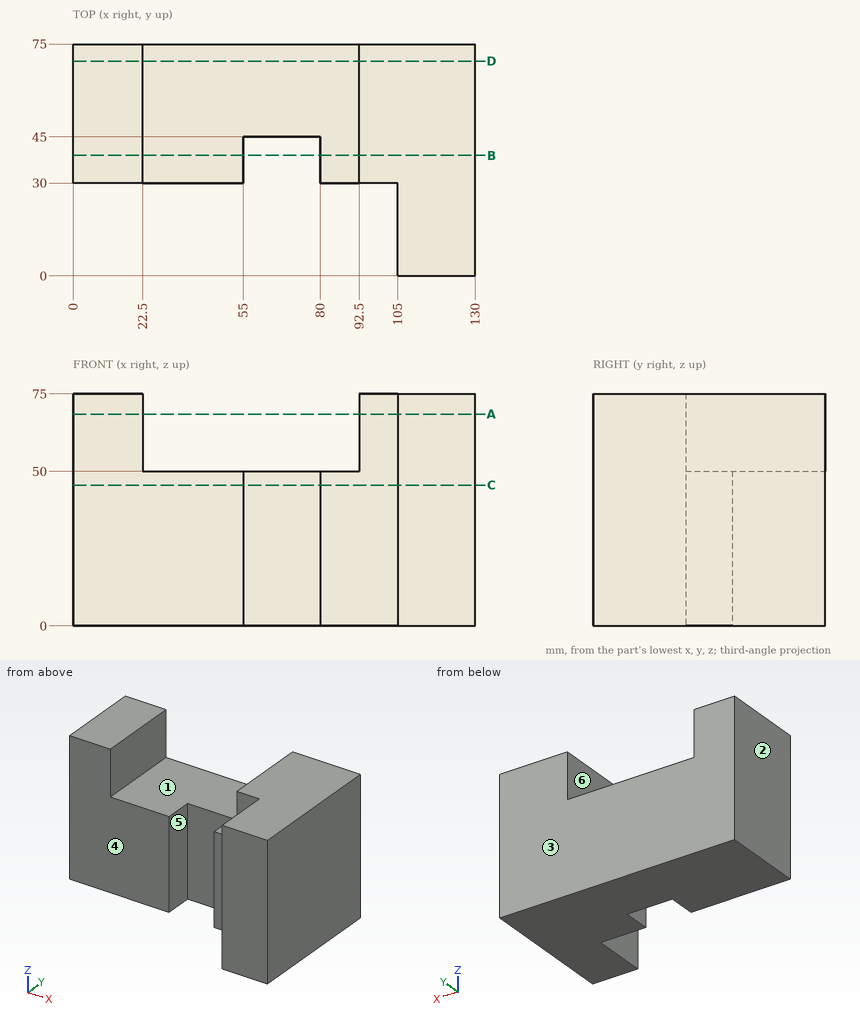
Study the drawing (mm; zero at the part's minimum x, y, z) and answer. A direction names the side the tool comes from. Round coordinates to 2 decimals unless told otherwise and drop trailing zeros. Write each loop counter-clockwise with the first axis right and the second up, starting at its lowest first coordinate (ties: lowest second). Pieces come first, ordered by that corner, then holes. Notation, with made-up numbers: (-29, -9) -> (-5, -9) arc R25 cw to (-5, 16) -> close; hole circle Ø3 at (9.5, -16.5). An arc over 180 degrees is marked (long way). Write each question's results on one line, items separated by ' | '.
Item 1: A cutting plane is placed at C-C, the plane z = 45.5. Determine the outline of the cut face in (x, y), plus the area to 4 significant figures.
Result set:
outline: (0, 30) -> (55, 30) -> (55, 45) -> (80, 45) -> (80, 30) -> (105, 30) -> (105, 0) -> (130, 0) -> (130, 75) -> (0, 75) -> close | area: 6,225 mm^2
Item 2: The mould has two halves that part along X. Classify the marked faces 1, 2 and 3: +X half, -X half, draft (parallel to the pull), parting line (faces both ways), or undercut.
Result set:
face 1: undercut | face 2: -X half | face 3: draft
Item 3: Find the intervals of material crossed by line 1 along X through (y, z) = (47.5, 64.5); line 2 along X through (y, z) = (13.5, 33.5); line 3 along X through (y, z) = (41.5, 34), in increasing order. Write a range as [from, to].
Result set:
line 1: [0, 22.5], [92.5, 130] | line 2: [105, 130] | line 3: [0, 55], [80, 130]
Item 4: A cutting plane is placed at A-A, the plane z = 68.5. Determine the outline of the cut face in (x, y).
Result set:
outline: (0, 30) -> (22.5, 30) -> (22.5, 75) -> (0, 75) -> close; (92.5, 30) -> (105, 30) -> (105, 0) -> (130, 0) -> (130, 75) -> (92.5, 75) -> close
Item 5: Which of the six approach directions +Z, -Z, +X, -X, +Y, -Y give full straight-line access (tool end or side, diameter ignored) to the marked faces 4, 5 and 6?
Result set:
face 4: +Z, -Z, -X, -Y | face 5: +Z, -Z, -Y | face 6: +Z, +Y, -Y
Item 6: Flat-ended cylindrical pins translate along their axes: P1, Ø3, axis at y = 42.5, z = 62.5, coming from the -X side; P2, Ø9, axis at y = 15, z = 32.5, coming from the -X side; P3, Ø20, axis at x = 68, z = 21, coming from the -Y side; P4, Ø7.5, axis at x = 90.5, z = 24.5, coming from the -Y side. Find the tip coordinate at first contact, or state that the pin passes through.
Result set:
P1: x = 0 | P2: x = 105 | P3: y = 45 | P4: y = 30
Item 7: A cutting plane is placed at D-D, the plane y = 69.5. Determine the outline of the cut face in (x, z), plus the area to 3 significant figures.
Result set:
outline: (0, 0) -> (130, 0) -> (130, 75) -> (92.5, 75) -> (92.5, 50) -> (22.5, 50) -> (22.5, 75) -> (0, 75) -> close | area: 8,000 mm^2
Item 8: A cutting plane is placed at B-B, the plane y = 39. Determine the outline of the cut face in (x, z).
Result set:
outline: (0, 0) -> (55, 0) -> (55, 50) -> (22.5, 50) -> (22.5, 75) -> (0, 75) -> close; (80, 0) -> (130, 0) -> (130, 75) -> (92.5, 75) -> (92.5, 50) -> (80, 50) -> close
